For this review, take the finished solid that the model builds, in its own axes (mm). Face numbers are marked on the shaded views. A direction names the side the tool comes from. Coordinates: 2 decimals unless noted, no trailing zeros. Write each loop counter-clockwise with the first axis right and the second up, starting at its lowest first coordinate (ties: lowest second). Pieces come first, ordered by that corner, then holes. Notation, with made-up numbers: (-15, 35.25) -> (20, 35.25) arc R25 ccw to (20, 53.25) -> close; hole circle Ø9 at (11, -40). An arc over 180 degrees is marked (long way). One line per item, written item: value. Start each with the question number.
1) Machinability: for the marked faces 3 and 4, which of the approach directions +Z, -Z, +X, -X, +Y, -Y give a long, thin tool a straight path to every point of the face, cutting with its end or side? Answer none if there is none.
2) Add section A-A (z = 0). State how many separate pieces and enclosed holes the cut face has, and give its area (3 significant figures).
3) Add section D-D (x = 7). State the section outline as (y, z) points, and give its area (4 significant figures).
4) Mouldability with a two-part tool opening along X and no side actions: class the marked faces 1 and 2 as released by +X, released by -X, zero draft, split by the parting line, or undercut.
5) Add section B-B (y = 2.1). State the section outline as (x, z) points.
6) For pin 1 Ø1.6 at (x, z) = (15, 0) entering from -Y; pin 2 Ø0.8 at (x, y) = (-9, 1.5) entering from -Z, all flat-tipped, find the tip position at first contact; note any pin that passes through.
7) Add section C-C (x = 15). State the section outline as (y, z) points, and give its area (3 significant figures).
8) For probe 1 along X at (y, z) = (1.8, 0); probe 2 along X at (y, z) = (1.5, 0.4); probe 3 along Z at (x, y) = (6.5, 0.55), list the stretches that pass through material, from the lowest coordinate up. Write a range as from..to.
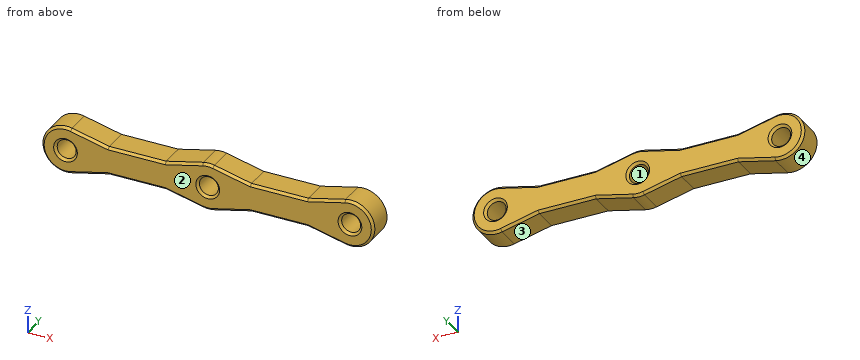
from build123d import *

# Parameters (mm, degrees)
SKETCH_1_R      = 1
EXTRUDE_1_DEPTH = 3
EXTRUDE_2_DEPTH = 3
CHAMFER_1_SIZE  = 0.25


with BuildPart() as part:
    # 草图1 → 凸台-拉伸1 (new body)
    with BuildSketch(Plane(origin=(0, 0, 0), x_dir=(1, 0, 0), z_dir=(0, 1, 0))):
        with BuildLine():
            Line((-13, 1.5), (-2, 1.5))
            ThreePointArc((-2, 1.5), (0, 2.5), (2, 1.5))
            Line((2, 1.5), (13, 1.5))
            ThreePointArc((13, 1.5), (17.5, 0), (13, -1.5))
            Line((13, -1.5), (2, -1.5))
            ThreePointArc((2, -1.5), (0, -2.5), (-2, -1.5))
            Line((-2, -1.5), (-13, -1.5))
            ThreePointArc((-13, -1.5), (-17.5, 0), (-13, 1.5))
        make_face()
        with Locations(Location((-15, 0, 0), (0, 0, 270))):
            Circle(SKETCH_1_R, mode=Mode.SUBTRACT)
        with Locations(Location((0, 0, 0), (0, 0, 270))):
            Circle(SKETCH_1_R, mode=Mode.SUBTRACT)
        with Locations(Location((15, 0, 0), (0, 0, 270))):
            Circle(SKETCH_1_R, mode=Mode.SUBTRACT)
    extrude(amount=EXTRUDE_1_DEPTH)

    # 草图2 → 凸台-拉伸2 (add)
    with BuildSketch(Plane(origin=(0, 0, 0), x_dir=(1, 0, 0), z_dir=(0, 1, 0))):
        with BuildLine():
            Line((4.5, 1.5), (0.578145188, 2.432231104))
            ThreePointArc((0.578145188, 2.432231104), (1.370755945, 2.090700395), (2, 1.5))
            Line((2, 1.5), (4.5, 1.5))
        make_face()
        with BuildLine():
            Line((4.5, -1.5), (0.578145188, -2.432231104))
            ThreePointArc((0.578145188, -2.432231104), (1.370755945, -2.090700395), (2, -1.5))
            Line((2, -1.5), (4.5, -1.5))
        make_face()
        with BuildLine():
            Line((10.5, 1.5), (14.421854812, 2.432231104))
            ThreePointArc((14.421854812, 2.432231104), (13.629244055, 2.090700395), (13, 1.5))
            Line((13, 1.5), (10.5, 1.5))
        make_face()
        with BuildLine():
            Line((10.5, -1.5), (14.421854812, -2.432231104))
            ThreePointArc((14.421854812, -2.432231104), (13.629244055, -2.090700395), (13, -1.5))
            Line((13, -1.5), (10.5, -1.5))
        make_face()
        with BuildLine():
            Line((-4.5, 1.5), (-2, 1.5))
            ThreePointArc((-2, 1.5), (-1.370755945, 2.090700395), (-0.578145188, 2.432231104))
            Line((-0.578145188, 2.432231104), (-4.5, 1.5))
        make_face()
        with BuildLine():
            Line((-10.5, -1.5), (-13, -1.5))
            ThreePointArc((-13, -1.5), (-13.629244055, -2.090700395), (-14.421854812, -2.432231104))
            Line((-14.421854812, -2.432231104), (-10.5, -1.5))
        make_face()
        with BuildLine():
            Line((-13, 1.5), (-10.5, 1.5))
            Line((-10.5, 1.5), (-14.421854812, 2.432231104))
            ThreePointArc((-14.421854812, 2.432231104), (-13.629244055, 2.090700395), (-13, 1.5))
        make_face()
        with BuildLine():
            Line((-2, -1.5), (-4.5, -1.5))
            Line((-4.5, -1.5), (-0.578145188, -2.432231104))
            ThreePointArc((-0.578145188, -2.432231104), (-1.370755945, -2.090700395), (-2, -1.5))
        make_face()
    extrude(amount=EXTRUDE_2_DEPTH)

    # 倒角1
    chamfer_1_edges = [part.edges().sort_by_distance(p)[0] for p in [
        (-7.5, 0, -1.5),
        (-7.5, 3, -1.5),
        (-2.539072594, 0, -1.966115552),
        (-2.539072594, 3, -1.966115552),
        (-15, 0, -1),
        (-15, 3, -1),
        (0, 0, -1),
        (0, 3, -1),
        (15, 0, -1),
        (15, 3, -1),
        (0, 0, -2.5),
        (0, 3, -2.5),
        (2.539072594, 0, -1.966115552),
        (2.539072594, 3, -1.966115552),
        (-17.5, 0, 0),
        (-17.5, 3, 0),
        (-12.460927406, 0, -1.966115552),
        (-12.460927406, 3, -1.966115552),
        (-7.5, 0, 1.5),
        (-7.5, 3, 1.5),
        (-12.460927406, 0, 1.966115552),
        (-12.460927406, 3, 1.966115552),
        (0, 0, 2.5),
        (0, 3, 2.5),
        (-2.539072594, 0, 1.966115552),
        (-2.539072594, 3, 1.966115552),
        (7.5, 0, 1.5),
        (7.5, 3, 1.5),
        (2.539072594, 0, 1.966115552),
        (2.539072594, 3, 1.966115552),
        (17.5, 0, 0),
        (17.5, 3, 0),
        (12.460927406, 0, 1.966115552),
        (12.460927406, 3, 1.966115552),
        (7.5, 0, -1.5),
        (7.5, 3, -1.5),
        (12.460927406, 0, -1.966115552),
        (12.460927406, 3, -1.966115552),
    ]]
    chamfer(chamfer_1_edges, length=CHAMFER_1_SIZE)


solid = part.part
Numbers:
1. face 3: -Z, +Y, -Y
1. face 4: +Y, -Y
2. separate pieces: 4
2. enclosed holes: 0
2. area: 86.5 mm²
3. outline: (0, -1.25) -> (0.25, -1.5) -> (2.75, -1.5) -> (3, -1.25) -> (3, 1.25) -> (2.75, 1.5) -> (0.25, 1.5) -> (0, 1.25) -> close
3. area: 8.875 mm²
4. face 1: undercut
4. face 2: zero draft
5. outline: (-14.42, -2.43) -> (-10.5, -1.5) -> (-4.5, -1.5) -> (-0.58, -2.43) arc R2.5 ccw to (0.58, -2.43) -> (4.5, -1.5) -> (10.5, -1.5) -> (14.42, -2.43) arc R2.5 ccw (long way) to (14.42, 2.43) -> (10.5, 1.5) -> (4.5, 1.5) -> (0.58, 2.43) arc R2.5 ccw to (-0.58, 2.43) -> (-4.5, 1.5) -> (-10.5, 1.5) -> (-14.42, 2.43) arc R2.5 ccw (long way) to start; hole circle Ø2 at (-15, 0); hole circle Ø2 at (0, 0); hole circle Ø2 at (15, 0)
6. pin 1: through
6. pin 2: z = -1.5
7. outline: (0, -2.25) -> (0.25, -2.5) -> (2.75, -2.5) -> (3, -2.25) -> (3, -1.25) -> (2.75, -1) -> (0.25, -1) -> (0, -1.25) -> close; (0, 1.25) -> (0.25, 1) -> (2.75, 1) -> (3, 1.25) -> (3, 2.25) -> (2.75, 2.5) -> (0.25, 2.5) -> (0, 2.25) -> close
7. area: 8.75 mm²
8. probe 1: -17.5..-16, -14..-1, 1..14, 16..17.5
8. probe 2: -17.47..-15.92, -14.08..-0.92, 0.92..14.08, 15.92..17.47
8. probe 3: -1.5..1.5
